Could you check a few things on this model? Use its own coordinates, in mm. Face numbers are marked on the shaded views. A direction names the side the tool comes from. Give positions to 0.01 mm unless a question says otherwise; leave off trailing zeros. Order: outer loops, then holes, each group sorted by start corner. A loop starts at its lowest first (then second) coordinate and runs counter-clockwise, first axis right, second up.
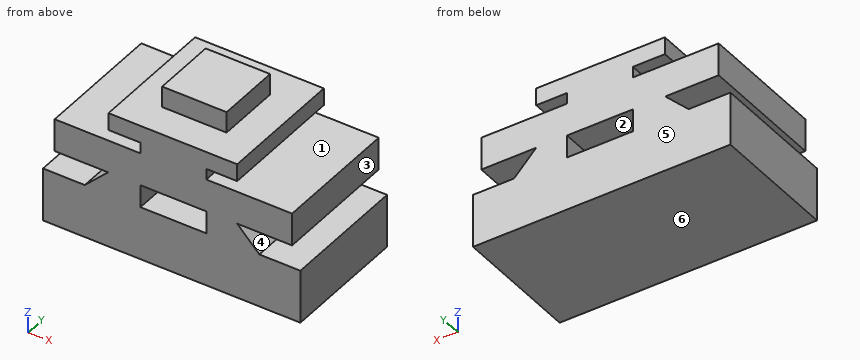
from build123d import *

# Parameters (mm, degrees)
F0_W     = 63.306741
F0_H     = 38.786522
F0_W_2   = 65.090016
F1_DEPTH = 76.2
F2_W     = 76.3532
F2_H     = 76.556332
F3_DEPTH = 101.6


with BuildPart() as f1:
    # F0 (on Front) → F1 (new body, symmetric)
    with BuildSketch(Plane.XZ):
        Polygon((-153.808624, -22.291109), (-153.808624, -85.597843), (151.133701, -85.597843), (151.133701, -22.291109), (102.539085, -22.291109), (39.678164, -22.291109), (-38.340699, -22.291109), (-104.322366, -22.291109), align=None)
        Polygon((-76.681398, 4.458224), (-104.322366, -22.291109), (-38.340699, -22.291109), (-38.340699, 4.458224), align=None)
        Polygon((39.678164, -22.291109), (102.539085, -22.291109), (76.235577, 4.458224), (39.678164, 4.458224), align=None)
        Polygon((-76.681398, 43.244746), (-76.681398, 4.458224), (-38.340699, 4.458224), (0, 4.458224), (0, 43.244746), (-38.340699, 43.244746), align=None)
        with Locations((-108.334768, 23.851485)):
            Rectangle(F0_W, F0_H)
        with Locations((108.780585, 23.851485)):
            Rectangle(F0_W_2, F0_H)
        Polygon((39.678164, 4.458224), (76.235577, 4.458224), (76.235577, 43.244746), (39.678164, 43.244746), (0, 43.244746), (0, 4.458224), align=None)
        Polygon((-38.340699, 56.173585), (-38.340699, 43.244746), (0, 43.244746), (39.678164, 43.244746), (39.678164, 56.173585), align=None)
        Polygon((-76.235577, 56.173585), (-38.340699, 56.173585), (39.678164, 56.173585), (76.235577, 56.173585), (76.235577, 76.681405), (-76.235577, 76.681405), align=None)
    extrude(amount=F1_DEPTH, both=True)

    # F2 (on Top) → F3 (join)
    with BuildSketch(Plane.XY):
        Rectangle(F2_W, F2_H)
    extrude(amount=F3_DEPTH)


solid = f1.part
Item 1: Imagine slicing it at D-D on z = -13. List the corners of the cut face in (x, y) for me, then the cut area to 3 significant figures.
Findings:
outline: (-94.72, -76.2) - (-38.34, -76.2) - (-38.34, 76.2) - (-94.72, 76.2) - close; (39.68, -76.2) - (93.4, -76.2) - (93.4, 76.2) - (39.68, 76.2) - close
area: 16,800 mm2
Item 2: Imagine slicing it at B-B on y = -55. List the corners of the cut face in (x, z) for me, then the cut area to 3 significant figures.
Findings:
outline: (-153.81, -85.6) - (151.13, -85.6) - (151.13, -22.29) - (102.54, -22.29) - (76.24, 4.46) - (141.33, 4.46) - (141.33, 43.24) - (39.68, 43.24) - (39.68, 56.17) - (76.24, 56.17) - (76.24, 76.68) - (-76.24, 76.68) - (-76.24, 56.17) - (-38.34, 56.17) - (-38.34, 43.24) - (-139.99, 43.24) - (-139.99, 4.46) - (-76.68, 4.46) - (-104.32, -22.29) - (-153.81, -22.29) - close; hole (-38.34, -22.29) - (39.68, -22.29) - (39.68, 4.46) - (-38.34, 4.46) - close
area: 37,100 mm2
Item 3: We'd pull the mould along Z, two halves only. Please class the marked faces 4, 5 and 6: +Z half, -Z half, draft (parallel to the pull), parting line (faces both ways), or undercut.
Findings:
face 4: undercut
face 5: draft
face 6: -Z half
Item 4: For the marked faces 1, 2 and 3, which set-ups out of +Z, -Z, +X, -X, +Y, -Y let a thin tool reach every point of the face, with its end or its side?
Findings:
face 1: +X, +Y, -Y
face 2: none
face 3: +Z, +X, +Y, -Y
Item 5: Imagine slicing it at C-C on x = 70. List the corners of the cut face in (y, z) for me, then the cut area to 3 significant figures.
Findings:
outline: (-76.2, -85.6) - (76.2, -85.6) - (76.2, 43.24) - (-76.2, 43.24) - close; (-76.2, 56.17) - (76.2, 56.17) - (76.2, 76.68) - (-76.2, 76.68) - close
area: 22,800 mm2
Item 6: Imagine slicing it at A-A on x = -28. List the corners of the cut face in (y, z) for me, then the cut area to 3 significant figures.
Findings:
outline: (-76.2, -85.6) - (76.2, -85.6) - (76.2, -22.29) - (-76.2, -22.29) - close; (-76.2, 4.46) - (-38.28, 4.46) - (-38.28, 0) - (38.28, 0) - (38.28, 4.46) - (76.2, 4.46) - (76.2, 76.68) - (38.28, 76.68) - (38.28, 101.6) - (-38.28, 101.6) - (-38.28, 76.68) - (-76.2, 76.68) - close
area: 22,900 mm2
Item 7: For pin 1 (14 mm diameter, centred on y = -31.5, z = 48, fed in from -X); pin 2 (2 mm diameter, centred on y = -36.5, z = 68.5, fed in from -X); pin 3 (4 mm diameter, centred on y = 35, z = -9.5, fed in from +X), each with a flat end and sliding along its axis, tell me the tip position at first contact or that it passes through.
Findings:
pin 1: stops at x = -139.99
pin 2: stops at x = -76.24
pin 3: stops at x = 91.93
Item 8: Please list where these lines run through material, in increasing order: line 1 along Z through (x, y) = (-1.5, 50.5); line 2 along Z through (x, y) = (-59, -6.5); line 3 along X through (y, z) = (15, 40.5).
Findings:
line 1: z = -85.6 to -22.29, 4.46 to 76.68
line 2: z = -85.6 to 43.24, 56.17 to 76.68
line 3: x = -139.99 to 141.33
